Geometry: see drawing. Coordinates: mm, zero at the bounding-box minimum. A direction names the side the tool comes from. Round coordinates to 2 decimals unless told otherwise and drop trailing zeros. Write each loop counter-clockwise with the first axis right and the second up, starting at its lowest first coordinate (ties: lowest second). Pieces come first, ordered by that corner, then holes. Notation, with made-up numbers: M -12,20.25 L -5,20.25 A5 ccw -5,24.25 Z; hole C 39,60.5 d5. An arc over 180 degrees is marked long. Use a Markdown table: item, result.
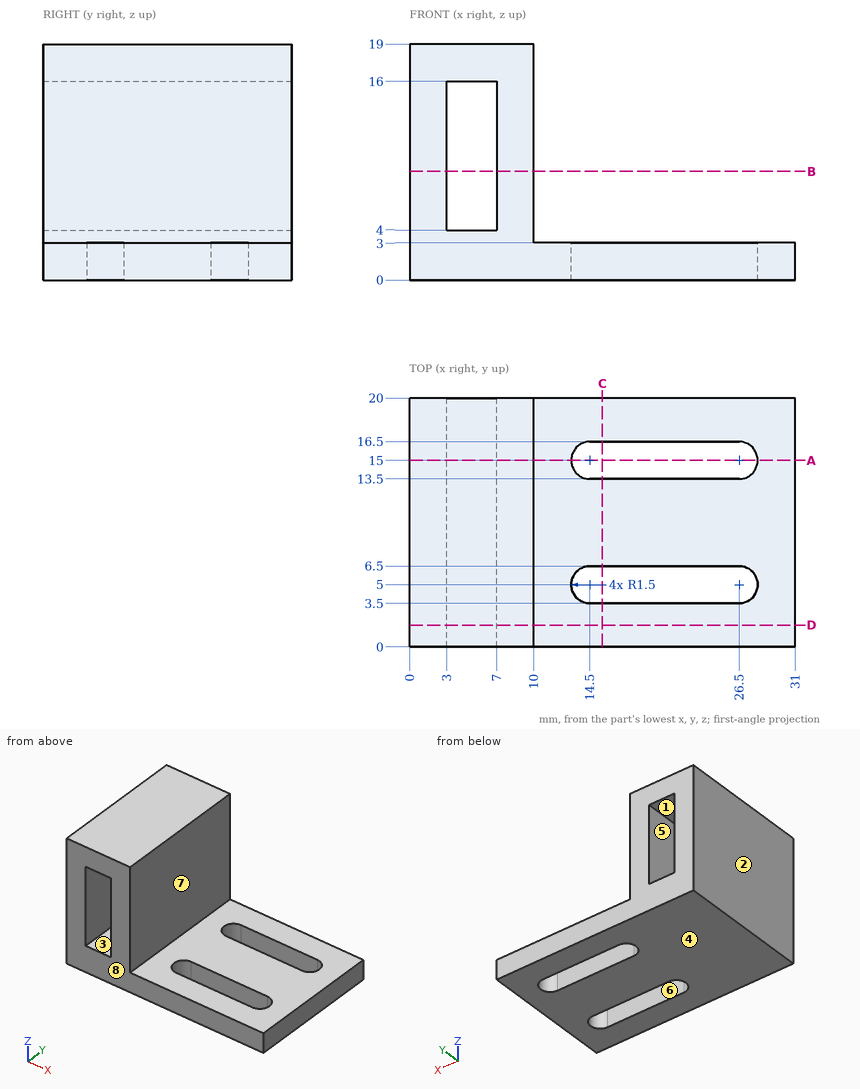
Q1. Section D-D on y = 1.75. Return loops of the section in (x, z).
Results are:
| item | result |
|---|---|
| outline | M 0,0 L 31,0 L 31,3 L 10,3 L 10,19 L 0,19 Z; hole M 3,4 L 7,4 L 7,16 L 3,16 Z |
Q2. First-contact query: pin 1 Ø6 at (x, y) = (21, 13.5) entering from +Z. Flat tip, straight axial feed; report the tip coordinate or a pass-through.
Results are:
| item | result |
|---|---|
| pin 1 | z = 3 |
Q3. Section C-C on x = 15.5. Return loops of the section in (y, z), plus the area to 3 significant figures.
Results are:
| item | result |
|---|---|
| outline | M 0,0 L 3.5,0 L 3.5,3 L 0,3 Z; M 6.5,0 L 13.5,0 L 13.5,3 L 6.5,3 Z; M 16.5,0 L 20,0 L 20,3 L 16.5,3 Z |
| area | 42.0 mm^2 |
Q4. Line query: L1, parallel to Y at x = 25.5, z = 1; L2, parallel to Z at x = 5, y = 13.75; L3, parallel to X at y = 12.5, z = 15.75. Output: solid intervals per line, ascending.
Results are:
| item | result |
|---|---|
| L1 | 0 to 3.5, 6.5 to 13.5, 16.5 to 20 |
| L2 | 0 to 4, 16 to 19 |
| L3 | 0 to 3, 7 to 10 |
Q5. Mould query, pull axis Z, two halves, no side actions, for the marked faces 1, 2, 3 and 4. Classes: +Z half, -Z half, draft (parallel to the pull), parting line (faces both ways), or undercut.
Results are:
| item | result |
|---|---|
| face 1 | undercut |
| face 2 | draft |
| face 3 | undercut |
| face 4 | -Z half |
Q6. Reachability of the marked faces 5, 6, 7 and 8 from +Z, -Z, +X, -X, +Y, -Y: full face, straight path, thin tool, end or side. Return the list, or none.
Results are:
| item | result |
|---|---|
| face 5 | +Y, -Y |
| face 6 | +Z, -Z |
| face 7 | +Z, +X, +Y, -Y |
| face 8 | +Z, -Z, +X, -X, -Y |
Q7. Section A-A on y = 15. Return loops of the section in (x, z), plus the area to 3 significant figures.
Results are:
| item | result |
|---|---|
| outline | M 0,0 L 13,0 L 13,3 L 10,3 L 10,19 L 0,19 Z; M 28,0 L 31,0 L 31,3 L 28,3 Z; hole M 3,4 L 7,4 L 7,16 L 3,16 Z |
| area | 160 mm^2 |
Q8. Section B-B on z = 8.75. Return loops of the section in (x, y).
Results are:
| item | result |
|---|---|
| outline | M 0,0 L 3,0 L 3,20 L 0,20 Z; M 7,0 L 10,0 L 10,20 L 7,20 Z |
